from build123d import *

# Parameters (mm, degrees)
SKETCH_1_W          = 50
SKETCH_1_H          = 50
EXTRUDE_1_DEPTH     = 20
SKETCH_2_W          = 30
SKETCH_2_H          = 30
EXTRUDE_2_DEPTH     = 10
SKETCH_3_W          = 30.2
SKETCH_3_H          = 30.2
SKETCH_3_W_2        = 30
SKETCH_3_H_2        = 30
CUT_EXTRUDE_1_DEPTH = 15


with BuildPart() as part:
    # 草图1 → 凸台-拉伸1 (new body)
    with BuildSketch(Plane(origin=(0, 0, 0), x_dir=(0, 0, -1), z_dir=(1, 0, 0))):
        Rectangle(SKETCH_1_W, SKETCH_1_H)
    extrude(amount=EXTRUDE_1_DEPTH)

    # 草图2 → 凸台-拉伸2 (add)
    with BuildSketch(Plane(origin=(20, 0, 0), x_dir=(0, 0, -1), z_dir=(1, 0, 0))):
        Rectangle(SKETCH_2_W, SKETCH_2_H)
    extrude(amount=EXTRUDE_2_DEPTH)

    # 草图3 → 切除-拉伸1 (cut)
    with BuildSketch(Plane(origin=(30, 0, 0), x_dir=(0, 0, -1), z_dir=(1, 0, 0))):
        Rectangle(SKETCH_3_W, SKETCH_3_H)
        Rectangle(SKETCH_3_W_2, SKETCH_3_H_2, mode=Mode.SUBTRACT)
    extrude(amount=-CUT_EXTRUDE_1_DEPTH, mode=Mode.SUBTRACT)


solid = part.part
CAD build for the part. Positions are in the model's coordinates, mm. A direction names the side the tool comes from. Round coordinates to 2 decimals unless told otherwise and drop trailing zeros. Write each loop counter-clockwise with the first axis right and the second up, starting at its lowest first coordinate (ties: lowest second). Pieces come first, ordered by that corner, then holes. Notation, with made-up numbers: (71, 68.25) -> (87, 68.25) arc R9 cw to (87, 83.25) -> close; hole circle Ø4 at (-33, -18.5). An arc over 180 degrees is marked (long way). Answer as a JSON object with one key per item and string values.
(1) Pin check, flat tip, straight feed: P1, Ø10, axis at x = 25.5, z = -11.5, coming from the -Y side. Stop position of the tip, or through.
Reported:
{"P1": "stops at y = -15"}
(2) Two-plate mould, pull along Y, no slides. Class faces 1 (the face through (23, 15, 0)), 2 (the face through (30, 0, 0)), 3 (the face through (10, 25, 0)): +Y half, -Y half, draft (parallel to the pull), parting line (faces both ways), or undercut.
Reported:
{"face 1": "undercut", "face 2": "draft", "face 3": "+Y half"}
(3) Band-saw the part on D-D, the plane y = -21. List the corners of the cut face in (x, z).
Reported:
{"outline": "(0, -25) -> (20, -25) -> (20, 25) -> (0, 25) -> close"}
(4) Which spindle directions (+Z, -Z, +X, -X, +Y, -Y) get a long thin tool onto all of the face, cutting with end or side? Do faces 4 (the face through (23, -15, 0)), 5 (the face through (0, 0, 0)). Say none if no direction does.
Reported:
{"face 4": "+X", "face 5": "+Z, -Z, -X, +Y, -Y"}
(5) Probe probe 1 along X at (y, z) = (7.5, 21); probe 2 along Z at (x, y) = (20.5, 3.5). List the from-to ranges inside material, lowest first. Write a range as [from, to].
Reported:
{"probe 1": "x = [0, 20]", "probe 2": "z = [-15, 15]"}
(6) Band-saw the part on A-A, the plane y = 7. List the corners of the cut face in (x, z).
Reported:
{"outline": "(0, -25) -> (20, -25) -> (20, -15.1) -> (15, -15.1) -> (15, -15) -> (30, -15) -> (30, 15) -> (15, 15) -> (15, 15.1) -> (20, 15.1) -> (20, 25) -> (0, 25) -> close"}
(7) Band-saw the part on C-C, the plane x = 27. List the corners of the cut face in (y, z).
Reported:
{"outline": "(-15, -15) -> (15, -15) -> (15, 15) -> (-15, 15) -> close"}
